```python
from build123d import *

# Parameters (mm, degrees)
SKETCH1_W                = 20
SKETCH1_H                = 40
SKETCH1_W_2              = 15
SKETCH1_H_2              = 15
SKETCH1_H_3              = 2.5
BOSS_EXTRUDE1_DEPTH      = 3
SKETCH2_W                = 5
SKETCH2_H                = 6.3
BOSS_EXTRUDE2_DEPTH      = 4
M3_CLEARANCE_HOLE1_D     = 3.6
M3_CLEARANCE_HOLE1_DEPTH = 10
M3_CLEARANCE_HOLE1_TIP   = 1.081549114
FILLET1_R                = 1.5


with BuildPart() as part:
    # Sketch1 → Boss-Extrude1 (new body)
    # profile 1 of 2: a face of its own
    with BuildSketch(Plane(origin=(0, 0, 0), x_dir=(1, 0, 0), z_dir=(0, 1, 0))):
        with Locations((10, 20)):
            Rectangle(SKETCH1_W, SKETCH1_H)
        with Locations((10, 30)):
            Rectangle(SKETCH1_W_2, SKETCH1_H_2, mode=Mode.SUBTRACT)
    # profile 2 of 2: a face of its own
    with BuildSketch(Plane(origin=(0, 0, 0), x_dir=(1, 0, 0), z_dir=(0, 1, 0))):
        with Locations((10, 30.25)):
            Rectangle(SKETCH1_W_2, SKETCH1_H_3)
    extrude(amount=BOSS_EXTRUDE1_DEPTH)

    # Sketch2 → Boss-Extrude2 (add)
    with BuildSketch(Plane(origin=(0, 3, 0), x_dir=(1, 0, 0), z_dir=(0, 1, 0))):
        with Locations((2.5, 10)):
            Rectangle(SKETCH2_W, SKETCH2_H)
        with Locations((17.5, 10)):
            Rectangle(SKETCH2_W, SKETCH2_H)
    extrude(amount=BOSS_EXTRUDE2_DEPTH)

    # M3 Clearance Hole1
    with Locations(Plane(origin=(0, 3, 0), x_dir=(1, 0, 0), z_dir=(0, 1, 0))):
        with Locations((10, 10)):
            Hole(M3_CLEARANCE_HOLE1_D / 2, depth=M3_CLEARANCE_HOLE1_DEPTH)
            with Locations((0, 0, -(M3_CLEARANCE_HOLE1_DEPTH + M3_CLEARANCE_HOLE1_TIP / 2))):  # 118° drill point
                Cone(0, M3_CLEARANCE_HOLE1_D / 2, M3_CLEARANCE_HOLE1_TIP, mode=Mode.SUBTRACT)

    # Fillet1
    fillet1_edges = [part.edges().sort_by_distance(p)[0] for p in [
        (2.5, 1.5, -37.5),
        (2.5, 1.5, -22.5),
        (17.5, 1.5, -22.5),
        (17.5, 1.5, -37.5),
        (0, 1.5, 0),
        (0, 1.5, -40),
        (20, 1.5, -40),
        (20, 1.5, 0),
        (2.5, 1.5, -31.5),
        (2.5, 1.5, -29),
        (17.5, 1.5, -31.5),
        (17.5, 1.5, -29),
    ]]
    fillet(fillet1_edges, radius=FILLET1_R)


solid = part.part
```
Geometry check sheet. Reference: the model listing, model coordinates, mm. A direction names the side the tool comes from. Give positions to 0.01 mm unless a question says otherwise; leave off trailing zeros. Order: outer loops, then holes, each group sorted by start corner. A loop starts at its lowest first (then second) coordinate and runs counter-clockwise, first axis right, second up.
1. Release check for a two-part mould opening along X. For faces 1 (the face through (2.95, 1.52, -31.93)), 2 (the face through (19.55, 1.52, -39.57)), 3 (the face through (2.5, 1, -26)), 4 (the face through (17, 5, -13.15)) record: pulls with the +X half, pulls with the -X half, needs draft (parallel to the pull), parting line crosses it, or undercut.
2. Section check C-C, the plane z = -27. Enter the section's corners in (x, y).
3. Section check B-B, the plane x = 10. Enter the section's corners in (y, z), and give its area (3 significant figures).
4. Section check A-A, the plane z = -10. Enter the section's corners in (x, y).
5. Thickness scan on L1, parallel to Z at x = 10, y = 2.3; L2, parallel to Z at x = 8, y = 1.5; L3, parallel to X at y = 1.05, z = -10. Record the ranges inside material, lowest first.
6. Gauge pin test, flat ends, axial feed: pin 1 Ø1.5 at (x, y) = (16, 5) entering from +Z; pin 2 Ø2 at (x, y) = (2, 5.5) entering from -Z; pin 3 Ø3 at (x, z) = (8.5, -23.5) entering from +Y. Record the tip position at first contact, or that the pin passes through.
7. Access from +Z, -Z, +X, -X, +Y, -Y to the whole of each face (thin tool, end or side, straight path). Record for faces 5 (the face through (2, 5, -13.15)), 6 (the face through (5, 5, -10)), 7 (the face through (10, 1, -29)).
8. Section check D-D, the plane z = -6. Enter the section's corners in (x, y).
Values follow:
1. face 1: undercut
1. face 2: pulls with the +X half
1. face 3: undercut
1. face 4: needs draft
2. outline: (0, 0) - (2.5, 0) - (2.5, 3) - (0, 3) - close; (17.5, 0) - (20, 0) - (20, 3) - (17.5, 3) - close
3. outline: (0, -40) - (3, -40) - (3, -37.5) - (0, -37.5) - close; (0, -31.5) - (3, -31.5) - (3, -29) - (0, -29) - close; (0, -22.5) - (3, -22.5) - (3, -11.8) - (0, -11.8) - close; (0, -8.2) - (3, -8.2) - (3, 0) - (0, 0) - close
3. area: 71.7 mm2
4. outline: (0, 0) - (8.2, 0) - (8.2, 3) - (5, 3) - (5, 7) - (0, 7) - close; (11.8, 0) - (20, 0) - (20, 7) - (15, 7) - (15, 3) - (11.8, 3) - close
5. L1: z = -40 to -37.5, -31.5 to -29, -22.5 to -11.8, -8.2 to 0
5. L2: z = -40 to -37.5, -31.5 to -29, -22.5 to 0
5. L3: x = 0 to 8.2, 11.8 to 20
6. pin 1: stops at z = -6.85
6. pin 2: stops at z = -13.15
6. pin 3: stops at y = 3
7. face 5: -Z, +X, -X, +Y
7. face 6: +Z, -Z, +Y
7. face 7: +Y, -Y
8. outline: (0, 0) - (20, 0) - (20, 3) - (0, 3) - close
